Geometry: see drawing. Coordinates: mm, zero at the bounding-box minimum. A direction names the side the tool comes from. Coordinates: 2 decimals unless noted, no trailing zeros. Write each loop counter-clockwise with the first axis right and the second up, starting at its lowest first coordinate (ties: lowest second). Pieces come first, ordered by that corner, then holes.
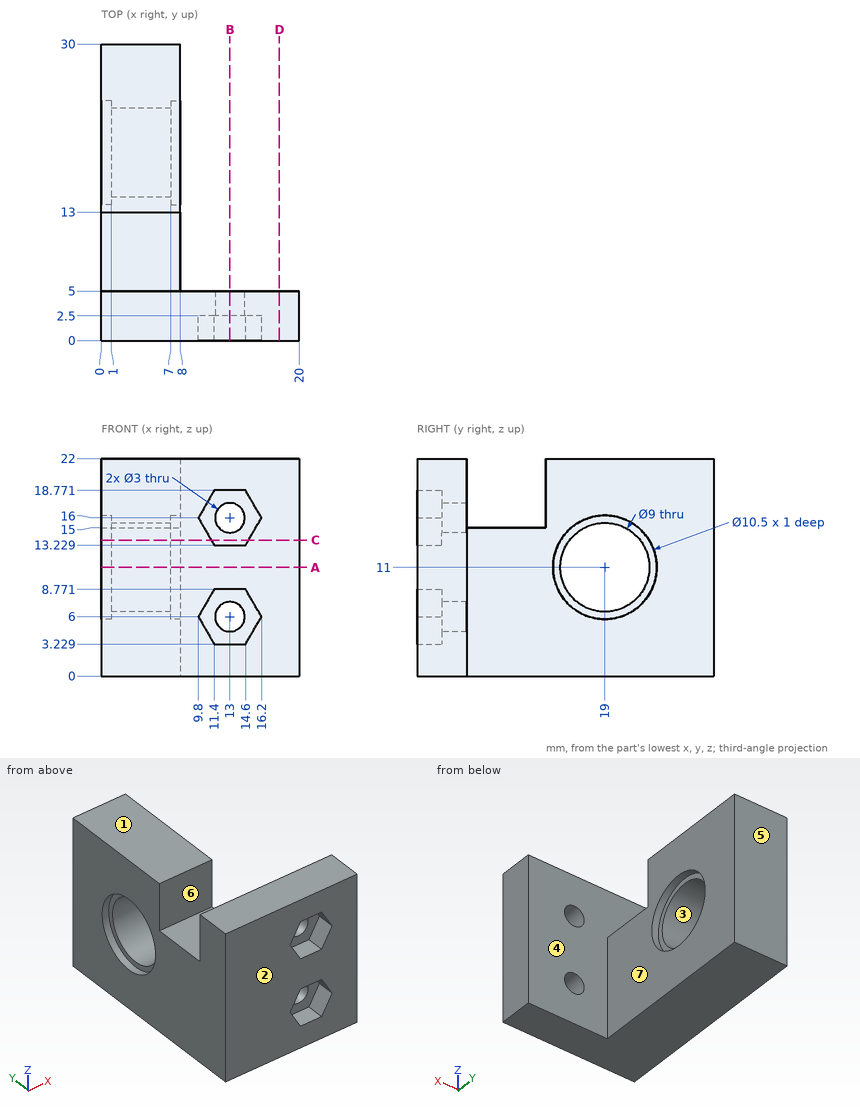
Item 1: Section D-D, the plane x = 18. Output: boundary loops of the cut face in (y, z).
Derived:
outline: (0, 0) - (5, 0) - (5, 22) - (0, 22) - close
Item 2: Pull-direction query (Y, two-part tool) for the marked faces 1, 2 and 3; classes: released by +Y, released by -Y, zero draft, split by the parting line, or undercut.
Derived:
face 1: zero draft
face 2: released by -Y
face 3: undercut
Item 3: Section B-B, the plane x = 13. Output: boundary loops of the cut face in (y, z), plus the area to 3 significant figures.
Derived:
outline: (0, 0) - (5, 0) - (5, 4.5) - (2.5, 4.5) - (2.5, 3.23) - (0, 3.23) - close; (0, 8.77) - (2.5, 8.77) - (2.5, 7.5) - (5, 7.5) - (5, 14.5) - (2.5, 14.5) - (2.5, 13.23) - (0, 13.23) - close; (0, 18.77) - (2.5, 18.77) - (2.5, 17.5) - (5, 17.5) - (5, 22) - (0, 22) - close
area: 67.3 mm2
Item 4: Material intervals for probe 1 along Z at (x, y) = (13, 3.8); probe 2 along Z at (x, y) = (3.5, 19.25); probe 3 along Y at (x, z) = (7.45, 11), sorted ascending.
Derived:
probe 1: z = 0 to 4.5, 7.5 to 14.5, 17.5 to 22
probe 2: z = 0 to 6.51, 15.49 to 22
probe 3: y = 0 to 13.75, 24.25 to 30
Item 5: Section C-C, the plane z = 13.75. Output: boundary loops of the cut face in (x, y).
Derived:
outline: (0, 0) - (11.1, 0) - (11.1, 2.5) - (14.9, 2.5) - (14.9, 0) - (20, 0) - (20, 5) - (8, 5) - (8, 14.53) - (7, 14.53) - (7, 15.44) - (1, 15.44) - (1, 14.53) - (0, 14.53) - close; (0, 23.47) - (1, 23.47) - (1, 22.56) - (7, 22.56) - (7, 23.47) - (8, 23.47) - (8, 30) - (0, 30) - close
Item 6: Section A-A, the plane z = 11. Output: boundary loops of the cut face in (x, y), plus the area to 3 significant figures.
Derived:
outline: (0, 0) - (20, 0) - (20, 5) - (8, 5) - (8, 13.75) - (7, 13.75) - (7, 14.5) - (1, 14.5) - (1, 13.75) - (0, 13.75) - close; (0, 24.25) - (1, 24.25) - (1, 23.5) - (7, 23.5) - (7, 24.25) - (8, 24.25) - (8, 30) - (0, 30) - close
area: 225 mm2
Item 7: Pin query (flat end, axial travel): pin 1 (11 mm diameter, centred on y = 13, z = 7, fed in from +X); pin 2 (3 mm diameter, centred on y = 17.5, z = 11.5, fed in from +X); pin 3 (2.5 mm diameter, centred on x = 5.5, y = 7.5, fed in from +Z); pin 4 (5 mm diameter, centred on x = 13, z = 6, fed in from -Y). Return the tip coordinate at first contact, or that it passes through.
Derived:
pin 1: stops at x = 8
pin 2: passes through
pin 3: stops at z = 15
pin 4: stops at y = 2.5
Item 8: Set-up query: the marked faces 4, 5, 6 and 7. Return all of +Z, -Z, +X, -X, +Y, -Y with unobstructed straight access to the full face (end or side cutting, diameter ignored); none if empty.
Derived:
face 4: +Z, +X
face 5: +Z, -Z, +X, -X, +Y
face 6: +Z, +X, -X
face 7: +Z, -Z, +X, +Y
